from build123d import *

# Parameters (mm, degrees)
EXTRUDE_3_DEPTH = 10
EXTRUDE_4_DEPTH = 20
EXTRUDE_5_DEPTH = 10
EXTRUDE_START   = 25
EXTRUDE_6_DEPTH = 25


with BuildPart() as part:
    # 草图1 → 凸台-拉伸3 (new body)
    with BuildSketch(Plane(origin=(0, 0, 0), x_dir=(1, 0, 0), z_dir=(0, 1, 0))):
        with BuildLine():
            Line((64.951905284, 37.5), (89.20061659, 51.5))
            ThreePointArc((89.20061659, 51.5), (99.490360108, 26.658361646), (103, 0))
            Line((103, 0), (75, 0))
            ThreePointArc((75, 0), (72.444436972, 19.411428383), (64.951905284, 37.5))
        make_face()
    extrude(amount=EXTRUDE_3_DEPTH)

    # 草图5 → 凸台-拉伸4 (add)
    with BuildSketch(Plane(origin=(0, 10, 0), x_dir=(1, 0, 0), z_dir=(0, 1, 0))):
        with BuildLine():
            Line((64.951905284, 37.5), (139.951905284, 37.5))
            Line((139.951905284, 37.5), (75, 0))
            ThreePointArc((75, 0), (72.444436972, 19.411428383), (64.951905284, 37.5))
        make_face()
    extrude(amount=EXTRUDE_4_DEPTH)

    # 草图6 → 凸台-拉伸5 (add)
    with BuildSketch(Plane(origin=(0, 30, 0), x_dir=(1, 0, 0), z_dir=(0, 1, 0))):
        Polygon((109.951905284, 37.5), (139.951905284, 37.5), (113.97114317, 22.5), align=None)
    extrude(amount=EXTRUDE_5_DEPTH)

    # 草图7 → 凸台-拉伸6 (add)
    with BuildSketch(Plane.XZ.offset(-10).offset(EXTRUDE_START)):
        with BuildLine():
            Line((89.20061659, -51.5), (91.798692801, -53))
            ThreePointArc((91.798692801, -53), (102.388137587, -27.434818781), (106, 0))
            Line((106, 0), (103, 0))
            ThreePointArc((103, 0), (99.490360108, -26.658361646), (89.20061659, -51.5))
        make_face()
    extrude(amount=-EXTRUDE_6_DEPTH)


solid = part.part
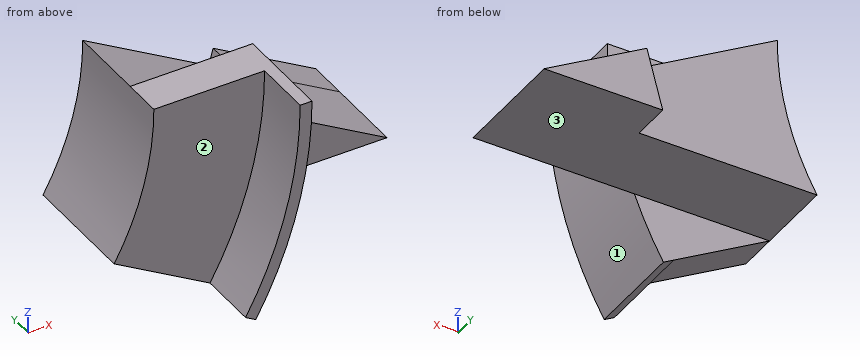
CAD build for the part. Positions are in the model's coordinates, mm. Face numbers are marked on the shaded views. A direction names the side the tool comes from. Round coordinates to 2 decimals unless told otherwise and drop trailing zeros. Order: outer loops, then holes, each group sorted by start corner. A loop starts at its lowest first (then second) coordinate and runs counter-clockwise, first axis right, second up. Notation, with made-up numbers: M 30.5,72 L 54.5,72 A23 cw 54.5,109 Z; hole C -18.75,48 d7. An arc over 180 degrees is marked long. Use one line per item in the form item = value.
Q1. Flat gauge pins, fed straight in: P1, Ø19, axis at x = 97.5, z = -23, coming from the +Y side; P2, Ø5, axis at y = 1, z = -10, coming from the +X side; P3, Ø24, axis at x = 84, y = 25.5, coming from the -Z side. Where does each tip first touch, or does it go through?
Recorded:
P1 = 30
P2 = 105.73
P3 = -37.5
Q2. Probe L1, parallel to Y at x = 81, z = -15.5; L2, parallel to Y at x = 125, z = -29.5; L3, parallel to X at y = 37, z = -32. List the from-to ranges inside material, lowest first.
Recorded:
L1 = 0 to 30
L2 = 10 to 40
L3 = 111.43 to 130.43
Q3. Saw through at A-A on x = 101. Give the cut face in (y, z), then the cut area to 3 significant figures.
Recorded:
outline = M -15,-32.17 L 10,-32.17 L 10,-37.5 L 30,-37.5 L 30,-15.01 L 10,-15.01 L 10,0 L 0,0 L 0,-20.2 L -15,-20.2 Z
area = 951 mm^2
Q4. Saw through at C-C on z = -42.5. Give the cut face in (x, y), then the cut area to 3 significant figures.
Recorded:
outline = M 73.61,0 L 93.82,0 L 93.82,-15 L 97.11,-15 L 97.11,10 L 73.61,10 Z
area = 284 mm^2
Q5. Which spindle directions (+Z, -Z, +X, -X, +Y, -Y) get a long thin tool onto all of the face, cutting with end or side? Do the marked faces 1, 2 and 3. Say none if no direction does.
Recorded:
face_1 = -Z, +X, -Y
face_2 = +Z, -X, -Y
face_3 = -Z, +X, -X, +Y
Q6. Saw through at D-D on x = 80. Give the cut face in (y, z), then the cut area to 3 significant figures.
Recorded:
outline = M 0,-46.19 L 10,-46.19 L 10,-37.5 L 30,-37.5 L 30,-2.89 L 10,-2.89 L 10,0 L 0,0 Z
area = 1,150 mm^2
Q7. Saw through at B-B on y = 9. Give the cut face in (x, z).
Recorded:
outline = M 64.95,-37.5 L 91.8,-53 A106 ccw 106,0 L 75,0 A75 cw Z
